Study the drawing (mm; zero at the part's minimum x, y, z) and answer. Round coordinates to 2 decimals unless told otherwise and drop trailing zeros. Write each loop counter-clockwise with the first axis right and the second up, starting at its lowest first coordinate (ties: lowest second). Pieces come first, ordered by that corner, then holes.
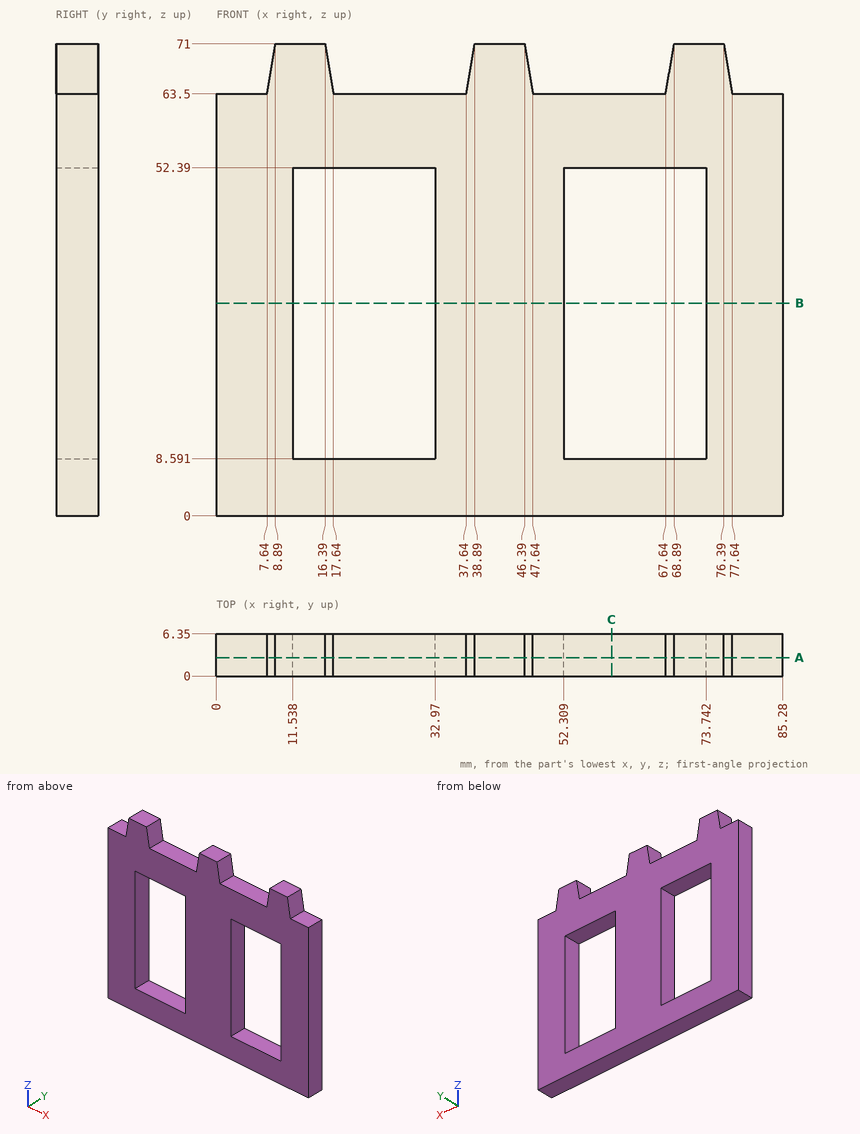
1. Straight lines are drawn through the part: line 1 along X through (y, z) = (1, 36); line 2 along Z through (x, y) = (23, 1.5); line 3 along Z through (x, y) = (35, 1.5). For each, find the intervals that lie inside material, in ascending order.
Geometry says:
line 1: x = 0 to 11.54, 32.97 to 52.31, 73.74 to 85.28
line 2: z = 0 to 8.59, 52.39 to 63.5
line 3: z = 0 to 63.5
2. Section B-B on z = 32 is taken. Determine the outline of the cut face in (x, y), plus the area to 3 significant figures.
Geometry says:
outline: (0, 0) - (11.54, 0) - (11.54, 6.35) - (0, 6.35) - close; (32.97, 0) - (52.31, 0) - (52.31, 6.35) - (32.97, 6.35) - close; (73.74, 0) - (85.28, 0) - (85.28, 6.35) - (73.74, 6.35) - close
area: 269 mm2
3. Section A-A on y = 2.75 is taken. Determine the outline of the cut face in (x, z).
Geometry says:
outline: (0, 0) - (85.28, 0) - (85.28, 63.5) - (77.64, 63.5) - (76.39, 71) - (68.89, 71) - (67.64, 63.5) - (47.64, 63.5) - (46.39, 71) - (38.89, 71) - (37.64, 63.5) - (17.64, 63.5) - (16.39, 71) - (8.89, 71) - (7.64, 63.5) - (0, 63.5) - close; hole (11.54, 8.59) - (32.97, 8.59) - (32.97, 52.39) - (11.54, 52.39) - close; hole (52.31, 8.59) - (73.74, 8.59) - (73.74, 52.39) - (52.31, 52.39) - close
4. Given pin 1 (1.9 mm diameter, centred on x = 66.5, y = 4.5, fed in from +Z), flat-ended and moving along its own axis, determine where the tip first touches the part or whether it passes through.
Geometry says:
pin 1: stops at z = 63.5
5. Section C-C on x = 59.5 is taken. Determine the outline of the cut face in (y, z).
Geometry says:
outline: (0, 0) - (6.35, 0) - (6.35, 8.59) - (0, 8.59) - close; (0, 52.39) - (6.35, 52.39) - (6.35, 63.5) - (0, 63.5) - close
